Autodesk Inventor part; units mm, degrees
ref_plane "YZ Plane" through (0, 0, 0) normal (1, 0, 0) x (0, 1, 0)
ref_plane "XZ Plane" through (0, 0, 0) normal (0, 1, 0) x (-1, 0, 0)
ref_plane "XY Plane" through (0, 0, 0) normal (0, 0, 1) x (1, 0, 0)
sketch "Sketch1" plane through (0, 0, 0) normal (0, 1, 0) x (-1, 0, 0)
  circle A0 centre (-37.3734, -58.1709) radius 1.5
  circle A1 centre (112.6266, 30.8291) radius 1.5
  circle A2 centre (-37.3734, 30.8291) radius 1.5
  circle A3 centre (112.6266, -58.1709) radius 1.5
  circle A4 centre (54.1266, -16.9209) radius 2.5
  circle A5 centre (-53.8734, 17.0791) radius 2.5
  circle A6 centre (54.1266, 17.0791) radius 2.5
  circle A7 centre (-53.8734, -16.9209) radius 2.5
  line L0 (-127.3734, 73.8291) -> (127.6266, 73.8291)
  line L1 (-127.3734, -73.6709) -> (-127.3734, 73.8291)
  line L2 (127.6266, -73.6709) -> (-127.3734, -73.6709)
  line L3 (127.6266, 73.8291) -> (127.6266, -73.6709)
  point P0 (0, 0)
  point P1 (0.1266, 73.8291)
extrude "Extrusion1" add sketch "Sketch1" along normal blind 10
sketch "Sketch2" plane through (127.3734, 0, 73.8291) normal (1, 0, 0) x (0, 0, -1)
  line L0 (147.5, 0) -> (147.5, 10)
  line L1 (0, 0) -> (0, 10)
  circle A0 centre (127.5, 5) radius 1.5
  circle A1 centre (20, 5) radius 1.5
  point P0 (73.8291, 0)
  point P1 (0, 5)
  dimension "d2" = 20
  dimension "d3" = 20
  dimension "d4" = 3
  dimension "d5" = 3
extrude "Extrusion2" cut sketch "Sketch2" against normal blind 6
ref_plane "Work Plane1" through (-0.1266, 0, 73.8291) normal (1, 0, 0) x (0, 0, -1)
mirror "Mirror1" about plane through (-0.1266, 0, 73.8291) normal (1, 0, 0) of "Extrusion2"
sketch "Sketch3" plane through (-127.6266, 0, 73.8291) normal (0, 0, 1) x (1, 0, 0)
  line L0 (255, 10) -> (0, 10)
  line L1 (255, 0) -> (0, 0)
  line L2 (0, 0) -> (0, 10)
  line L3 (0, 10) -> (255, 10)
  line L4 (255, 10) -> (255, 0)
  point P0 (127.6266, 0)
extrude "Extrusion3" cut sketch "Sketch3" against normal blind 10
sketch "Sketch4" plane through (0, 10, 0) normal (0, 1, 0) x (1, 0, 0)
  line L0 (127.3734, -63.8291) -> (127.3734, 73.6709)
  line L1 (-127.6266, -63.8291) -> (127.3734, -63.8291)
  line L2 (127.3734, -63.8291) -> (127.3734, 73.6709)
  line L3 (127.3734, 73.6709) -> (-127.6266, 73.6709)
  line L4 (-127.6266, 73.6709) -> (-127.6266, -63.8291)
  point P0 (0, 0)
ref_plane "Work Plane2" through (0, 5, 0) normal (0, 1, 0) x (1, 0, 0)
extrude "Extrusion4" cut sketch "Sketch4" against normal blind 2.5
mirror "Mirror2" about plane through (0, 5, 0) normal (0, 1, 0) of "Extrusion4"
sketch "Sketch6" plane through (0, 7.5, 0) normal (0, 1, 0) x (1, 0, 0)
  circle A0 centre (37.3734, 58.1709) radius 1.5
  circle A1 centre (-112.6266, -30.8291) radius 1.5
  circle A2 centre (37.3734, -30.8291) radius 1.5
  circle A3 centre (-112.6266, 58.1709) radius 1.5
  circle A4 centre (-54.1266, 16.9209) radius 2.5
  circle A5 centre (53.8734, -17.0791) radius 2.5
  circle A6 centre (-54.1266, -17.0791) radius 2.5
  circle A7 centre (53.8734, 16.9209) radius 2.5
  line L0 (127.3734, 73.6709) -> (127.3734, -63.8291)
  line L1 (-127.6266, 73.6709) -> (127.3734, 73.6709)
  line L2 (-127.6266, -63.8291) -> (-127.6266, 73.6709)
  line L3 (127.3734, -63.8291) -> (-127.6266, -63.8291)
  line L4 (-30, 54.9209) -> (30, 54.9209)
  line L5 (30, 54.9209) -> (30, -45.0791)
  line L6 (30, -45.0791) -> (-30, -45.0791)
  line L7 (-30, -45.0791) -> (-30, 54.9209)
  line L8 (-105, 54.9209) -> (-65, 54.9209)
  line L9 (-65, 54.9209) -> (-65, -45.0791)
  line L10 (-65, -45.0791) -> (-105, -45.0791)
  line L11 (-105, -45.0791) -> (-105, 54.9209)
  line L12 (65, 54.9209) -> (105, 54.9209)
  line L13 (105, 54.9209) -> (105, -45.0791)
  line L14 (105, -45.0791) -> (65, -45.0791)
  line L15 (65, -45.0791) -> (65, 54.9209)
  line L16 (-65, 4.9209) -> (-30, 4.9209) construction
  line L17 (30, 4.9209) -> (65, 4.9209) construction
  line L18 (0, 0) -> (0, 54.9209) construction
  line L19 (0, 54.9209) -> (-0.1266, 73.6709) construction
  line L20 (0, -45.0791) -> (-0.1266, -63.8291) construction
  line L21 (-105, 54.9209) -> (-65, -45.0791) construction
  line L22 (-103.143, 55.6637) -> (-63.143, -44.3363)
  line L23 (-106.857, 54.1781) -> (-66.857, -45.8219)
  line L24 (-30, 54.9209) -> (30, -45.0791)
  line L25 (-31.715, 53.8919) -> (28.285, -46.1081)
  line L26 (-28.285, 55.9499) -> (31.715, -44.0501)
  line L27 (65, 54.9209) -> (105, -45.0791) construction
  line L28 (57.4212, 79.253) -> (105, -39.6939)
  line L29 (53.7073, 77.7675) -> (103.2874, -46.1827)
  point P0 (67.1541, 54.9209)
  point P1 (102.8459, -45.0791)
  point P2 (65, 49.5357)
  point P3 (-27.6676, 54.9209)
  point P4 (30, -41.1918)
  point P5 (27.6676, -45.0791)
  point P6 (-30, 51.0336)
  point P7 (-102.8459, 54.9209)
  point P8 (-65, -39.6939)
  point P9 (-67.1541, -45.0791)
  point P10 (-105, 49.5357)
  dimension "d12" = 60
  dimension "d13" = 100
  dimension "d14" = 40
  dimension "d15" = 35
  dimension "d16" = 2
  dimension "d17" = 2
  dimension "d18" = 2
  dimension "d19" = 2
  dimension "d20" = 2
  dimension "d21" = 2
extrude "Extrusion5" cut sketch "Sketch6" against normal through all contours L12 L13 L28 | L29 L14 L15 | L4 L5 L26 | L25 L6 L7 | L8 L9 L22 | L23 L10 L11
ref_plane "Work Plane3" through (0, 5, 0) normal (0, 1, 0) x (1, 0, 0)
equation "\"d17\" = d16"
equation "\"d18\" = d16"
equation "\"d19\" = d16"
equation "\"d20\" = d16"
equation "\"d21\" = d20"
properties part number "midplate_3DPrint"
The model under review builds one solid part; all positions refer to its coordinate system, in mm. A direction names the side the tool comes from. Give positions to 0.01 mm unless a question says otherwise; leave off trailing zeros. Loops run counter-clockwise (first coordinate to the right, second up) from the corner with the lowest first, then second, coordinate; pieces in that order, holes last. Notation, with made-up numbers: (68.5, -20) - (103.5, -20) arc R27 ccw to (103.5, 9) - close; hole circle Ø10 at (25.5, 29.25). An arc over 180 degrees is marked (long way). Answer as a JSON object with one key per item and string values.
Q1. Add section C-C on x = 70. State the section outline as (y, z) points, plus the area to 3 significant figures.
Worked out:
{"outline": "(2.5, -73.67) - (7.5, -73.67) - (7.5, -54.92) - (2.5, -54.92) - close; (2.5, -47.81) - (7.5, -47.81) - (7.5, -37.04) - (2.5, -37.04) - close; (2.5, 45.08) - (7.5, 45.08) - (7.5, 63.83) - (2.5, 63.83) - close", "area": "241 mm^2"}
Q2. Add section B-B on x = -21. State the section outline as (y, z) points, plus the area to 3 significant figures.
Worked out:
{"outline": "(2.5, -73.67) - (7.5, -73.67) - (7.5, -54.92) - (2.5, -54.92) - close; (2.5, -43.81) - (7.5, -43.81) - (7.5, -36.03) - (2.5, -36.03) - close; (2.5, 45.08) - (7.5, 45.08) - (7.5, 63.83) - (2.5, 63.83) - close", "area": "226 mm^2"}
Q3. Insertion check: pin 1 (3.5 mm diameter, centred on x = 37.37, z = -58.17, fed in from -Y); pin 2 (0.9 mm diameter, centred on y = 5, z = -54.5, fed in from +X). Each pin has a flat end and moves straight along its axis. Give the tip position at first contact, or say it passes through.
Worked out:
{"pin 1": "stops at y = 2.5", "pin 2": "stops at x = 121.37"}
Q4. To check wall thickness, follow line 1 along X through (y, z) = (4.1, -58); line 2 along Z through (x, y) = (79, 2.7); line 3 along Z through (x, y) = (72.5, 3.6). State the ranges of each line that lie inside material, in increasing order.
Worked out:
{"line 1": "x = -127.63 to -114.12, -111.14 to 35.88, 38.86 to 127.37", "line 2": "z = -73.67 to -54.92, -25.31 to -14.54, 45.08 to 63.83", "line 3": "z = -73.67 to -54.92, -41.56 to -30.79, 45.08 to 63.83"}
Q5. For faces 4 (the flat face through (65, 5, -2)), 5 (the flat face through (-127.627, 5, -4)), list the 3-axis set-ups (+Z, -Z, +X, -X, +Y, -Y) from which the entire face can be reached by the end or side of a thin tool; tool diameter is ignored.
Worked out:
{"face 4": "+Y, -Y", "face 5": "+Z, -Z, -X, +Y, -Y"}
Q6. Mouldability with a two-part tool opening along X and no side actions: class faces 1 (the flat face through (127.373, 5, -6)), 2 (the flat face through (-84, 5, -54.921)), 3 (the flat face through (-2, 5, -73.671)) as +X half, -X half, draft (parallel to the pull), parting line (faces both ways), or undercut.
Worked out:
{"face 1": "+X half", "face 2": "undercut", "face 3": "draft"}
Q7. Add section D-D on y = 5. Count the separate pieces of the cut face and the enclosed holes in it, plus the area to 3 significant figures.
Worked out:
{"separate pieces": "1", "enclosed holes": "14", "area": "22,200 mm^2"}
Q8. Add section A-A on z = -3.5. State the section outline as (x, y) points.
Worked out:
{"outline": "(-127.63, 2.5) - (-105, 2.5) - (-105, 7.5) - (-127.63, 7.5) - close; (-86.59, 2.5) - (-82.28, 2.5) - (-82.28, 7.5) - (-86.59, 7.5) - close; (-65, 2.5) - (-30, 2.5) - (-30, 7.5) - (-65, 7.5) - close; (-1.48, 2.5) - (3.18, 2.5) - (3.18, 7.5) - (-1.48, 7.5) - close; (30, 2.5) - (65, 2.5) - (65, 7.5) - (30, 7.5) - close; (83.41, 2.5) - (87.72, 2.5) - (87.72, 7.5) - (83.41, 7.5) - close; (105, 2.5) - (127.37, 2.5) - (127.37, 7.5) - (105, 7.5) - close"}
